Here's how the part is built. I have some questions about the finished solid (model axes, mm). Coordinates: 2 decimals unless noted, no trailing zeros. Write each loop counter-clockwise with the first axis right and the second up, starting at its lowest first coordinate (ties: lowest second). Pieces come first, ordered by that corner, then holes. Notation, with made-up numbers: M -35.5,-14.5 L 10.5,-14.5 A13 cw 10.5,-7.5 Z; hole C 6,70 d10. An arc over 180 degrees is marked long. Use one line per item in the form item = value. Start each with the question number.
1. Please list where these lines run through material, in increasing order: line 1 along X through (y, z) = (149.5, 2.3); line 2 along X through (y, z) = (59, 1.95); line 3 along X through (y, z) = (114.5, 2.9). Write a range as [from, to].
2. I want a section at C-C, the plane x = -37. List the corners of the cut face in (y, z) for me, plus the area to 3 significant figures.
3. I want a section at A-A, the plane y = 127. Count the separate pieces of the cut face and the enclosed holes in it, plus the area to 3 significant figures.
4. I'm going to push flat-ended pins straight in: pin 1 Ø3 at (x, z) = (-80, 4) entering from +Y; pin 2 Ø2.5 at (x, y) = (-116.73, 68.75) entering from +Z; pin 3 Ø1 at (x, z) = (88, 4) entering from +Y; pin 4 Ø1.5 at (x, z) = (87.5, 3) entering from +Y. Where does each tip first touch, or does it pass through?
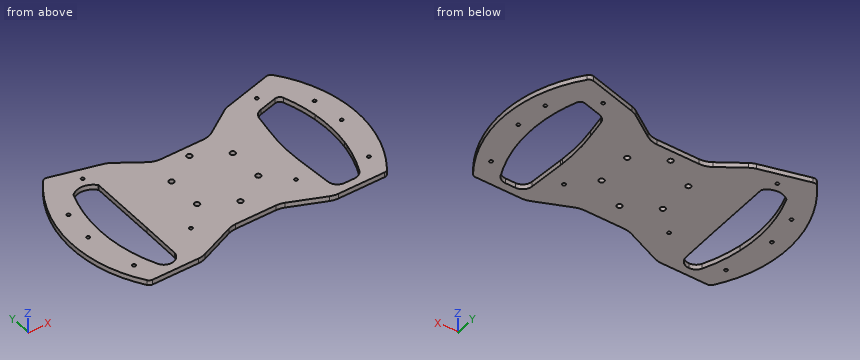
from build123d import *

# Parameters (mm, degrees)
SKETCH7_R           = 1.6
SKETCH7_R_2         = 2.55
BOSS_EXTRUDE2_DEPTH = 5


with BuildPart() as part:
    # Sketch7 → Boss-Extrude2 (new body)
    with BuildSketch(Plane(origin=(-155.165218795, 0, 0), x_dir=(1, 0, 0), z_dir=(0, 0, 1))):
        with BuildLine():
            ThreePointArc((186.769671741, 167.286880781), (181.433247766, 164.741537113), (175.585813672, 163.867632232))
            Line((175.585813672, 163.867632232), (133.81504093, 163.867632232))
            ThreePointArc((133.81504093, 163.867632232), (127.967606836, 164.741537113), (122.631182861, 167.286880781))
            Line((122.631182861, 167.286880781), (98.971665752, 183.245426575))
            ThreePointArc((98.971665752, 183.245426575), (96.081672536, 184.863900542), (92.964188585, 185.98319165))
            Line((92.964188585, 185.98319165), (46.183315852, 198.51808872))
            ThreePointArc((46.183315852, 198.51808872), (43.329318726, 198.438902311), (40.983947586, 196.81077323))
            ThreePointArc((40.983947586, 196.81077323), (13.687864292, 122.997631993), (35.910853464, 47.501971622))
            ThreePointArc((35.910853464, 47.501971622), (37.700666361, 45.921987917), (40.019050269, 45.352010045))
            Line((40.019050269, 45.352010045), (85.367161343, 45.352010045))
            ThreePointArc((85.367161343, 45.352010045), (89.354520031, 45.753515952), (93.181783913, 46.941912976))
            Line((93.181783913, 46.941912976), (126.95485072, 61.277729301))
            ThreePointArc((126.95485072, 61.277729301), (130.782114601, 62.466126325), (134.769473289, 62.867632232))
            Line((134.769473289, 62.867632232), (174.631381312, 62.867632232))
            ThreePointArc((174.631381312, 62.867632232), (178.618740001, 62.466126325), (182.446003882, 61.277729301))
            Line((182.446003882, 61.277729301), (216.219070689, 46.941912976))
            ThreePointArc((216.219070689, 46.941912976), (220.04633457, 45.753515952), (224.033693259, 45.352010045))
            Line((224.033693259, 45.352010045), (269.381804333, 45.352010045))
            ThreePointArc((269.381804333, 45.352010045), (271.70018824, 45.921987917), (273.490001138, 47.501971622))
            ThreePointArc((273.490001138, 47.501971622), (295.712990309, 122.997631993), (268.416907015, 196.81077323))
            ThreePointArc((268.416907015, 196.81077323), (266.071535876, 198.438902311), (263.217538749, 198.51808872))
            Line((263.217538749, 198.51808872), (216.436666017, 185.98319165))
            ThreePointArc((216.436666017, 185.98319165), (213.319182066, 184.863900542), (210.42918885, 183.245426575))
            Line((210.42918885, 183.245426575), (186.769671741, 167.286880781))
        make_face()
        with Locations((38.436607979, 68.752932179)):
            Circle(SKETCH7_R, mode=Mode.SUBTRACT)
        with Locations((102.700427301, 79.752932179)):
            Circle(SKETCH7_R, mode=Mode.SUBTRACT)
        with Locations((29.203576285, 118.752932179)):
            Circle(SKETCH7_R, mode=Mode.SUBTRACT)
        with BuildLine():
            ThreePointArc((50.870986739, 168.810905662), (63.047418465, 172.817129133), (74.292978733, 166.664675124))
            Line((74.292978733, 166.664675124), (74.292978733, 100.280747179))
            Line((74.292978733, 100.280747179), (73.980283138, 62.561010441))
            ThreePointArc((73.980283138, 62.561010441), (70.797263007, 56.006603452), (64.011616245, 53.352010045))
            ThreePointArc((64.011616245, 53.352010045), (58.655129241, 54.907600831), (54.965142603, 59.09040065))
            ThreePointArc((54.965142603, 59.09040065), (48.044160974, 76.816977425), (43.591061483, 95.318366989))
            ThreePointArc((43.591061483, 95.318366989), (42.297615396, 132.553323304), (50.870986739, 168.810905662))
        make_face(mode=Mode.SUBTRACT)
        with Locations((124.389538168, 101.252932179)):
            Circle(SKETCH7_R_2, mode=Mode.SUBTRACT)
        with Locations((206.700427301, 79.752932179)):
            Circle(SKETCH7_R, mode=Mode.SUBTRACT)
        with Locations((270.964246623, 68.752932179)):
            Circle(SKETCH7_R, mode=Mode.SUBTRACT)
        with Locations((154.700427301, 83.752932179)):
            Circle(SKETCH7_R_2, mode=Mode.SUBTRACT)
        with Locations((185.011316433, 101.252932179)):
            Circle(SKETCH7_R_2, mode=Mode.SUBTRACT)
        with BuildLine():
            Line((235.107875868, 167.174775102), (252.566315963, 171.852750026))
            ThreePointArc((252.566315963, 171.852750026), (256.132298182, 171.477167312), (258.529867862, 168.810905662))
            ThreePointArc((258.529867862, 168.810905662), (263.529184961, 153.009876594), (266.626244503, 136.728785929))
            add(Edge.make_bspline(
                [(266.626244503, 136.728785929), (269.27120455, 115.705359984), (265.809793118, 95.318366989)],
                knots=[0, 0, 0, 0.881934454, 0.881934454, 0.881934454], degree=2))
            ThreePointArc((265.809793118, 95.318366989), (265.318661666, 92.589710086), (264.773591938, 89.871313942))
            ThreePointArc((264.773591938, 89.871313942), (260.500059228, 74.180131562), (254.435711999, 59.09040065))
            ThreePointArc((254.435711999, 59.09040065), (250.745725361, 54.907600831), (245.389238357, 53.352010045))
            Line((245.389238357, 53.352010045), (235.807999121, 53.352010045))
            ThreePointArc((235.807999121, 53.352010045), (229.022352359, 56.006603452), (225.839332228, 62.561010441))
            Line((225.839332228, 62.561010441), (223.081153151, 97.32129138))
            add(Edge.make_bspline(
                [(222.846324523, 100.280747179), (222.950560925, 98.800835847), (223.081153151, 97.32129138)],
                knots=[0.931930938, 0.931930938, 0.931930938, 1, 1, 1], degree=2))
            add(Edge.make_bspline(
                [(224.932331274, 140.872333064), (221.419227915, 120.542156926), (222.846324523, 100.280747179)],
                knots=[0, 0, 0, 0.931930938, 0.931930938, 0.931930938], degree=2))
            Line((224.932331274, 140.872333064), (227.819439706, 159.081481956))
            ThreePointArc((227.819439706, 159.081481956), (230.265167007, 164.207432514), (235.107875868, 167.174775102))
        make_face(mode=Mode.SUBTRACT)
        with Locations((280.197278317, 118.752932179)):
            Circle(SKETCH7_R, mode=Mode.SUBTRACT)
        with Locations((32.909775986, 150.752932179)):
            Circle(SKETCH7_R, mode=Mode.SUBTRACT)
        with Locations((124.389538168, 136.252932179)):
            Circle(SKETCH7_R_2, mode=Mode.SUBTRACT)
        with Locations((68.540177705, 180.621909566)):
            Circle(SKETCH7_R, mode=Mode.SUBTRACT)
        with Locations((185.011316433, 136.252932179)):
            Circle(SKETCH7_R_2, mode=Mode.SUBTRACT)
        with Locations((154.700427301, 153.752932179)):
            Circle(SKETCH7_R_2, mode=Mode.SUBTRACT)
        with Locations((276.491078616, 150.752932179)):
            Circle(SKETCH7_R, mode=Mode.SUBTRACT)
        with Locations((240.860676897, 180.621909566)):
            Circle(SKETCH7_R, mode=Mode.SUBTRACT)
    extrude(amount=BOSS_EXTRUDE2_DEPTH)


solid = part.part
Answer list:
q1.line_1 = [-137.71, -123.25], [-121.26, -110.13], [-80.87, 71.14], [109.2, 120.33], [122.32, 136.78]
q1.line_2 = [-126.34, -100.16], [-82.15, -33.58], [32.65, 71.64], [99.23, 125.41]
q1.line_3 = [-141.48, -113.48], [-80.87, 67.29], [112.55, 140.55]
q2.outline = M 57.55,0 L 170.3,0 L 170.3,5 L 57.55,5 Z
q2.area = 564 mm²
q3.separate_pieces = 3
q3.enclosed_holes = 0
q3.area = 1,020 mm²
q4.pin_1 = 191.15
q4.pin_2 = through
q4.pin_3 = 193.28
q4.pin_4 = 193.21
